```python
from build123d import *

# Parameters (mm, degrees)
F1_DEPTH = 609.6
F2_R     = 12.7
F3_DEPTH = 406.401
F4_T     = -2.54
F5_R     = 12.7
F5_R_2   = 3.302
F6_DEPTH = 25.4


with BuildPart() as f1:
    # F0 (on Top) → F1 (new body)
    with BuildSketch(Plane.XY):
        with BuildLine():
            Line((203.2, -101.6), (203.2, 114.3))
            Line((203.2, 114.3), (-203.2, 114.3))
            Line((-203.2, 114.3), (-203.2, -101.6))
            ThreePointArc((-203.2, -101.6), (-194.2197438789, -105.3197438789), (-190.5, -114.3))
            Line((-190.5, -114.3), (190.5, -114.3))
            ThreePointArc((190.5, -114.3), (194.2197438789, -105.3197438789), (203.2, -101.6))
        make_face()
    extrude(amount=F1_DEPTH)

    # F2 (on face) → F3 (cut, through all)
    with BuildSketch(Plane.YZ.offset(203.2)):
        with Locations((-114.2978898402, 609.8315029268)):
            Circle(F2_R)
        with Locations((-114.3, 0)):
            Circle(F2_R)
    extrude(amount=-F3_DEPTH, mode=Mode.SUBTRACT)

    # F4
    f4_openings = [f1.faces().sort_by_distance(p)[0] for p in [
        (0, -114.3, 304.915752),
    ]]
    offset(amount=F4_T, openings=f4_openings)

    # F5 (on face) → F6 (cut)
    with BuildSketch(Plane.XY.offset(609.6)):
        with Locations((127, 25.4)):
            Circle(F5_R)
        with Locations((101.6, 25.4)):
            Circle(F5_R_2)
    extrude(amount=-F6_DEPTH, mode=Mode.SUBTRACT)


solid = f1.part
```
CAD build for the part. Positions are in the model's coordinates, mm. A direction names the side the tool comes from. Coordinates: 2 decimals unless noted, no trailing zeros. Loops run counter-clockwise (first coordinate to the right, second up) from the corner with the lowest first, then second, coordinate; pieces in that order, holes last. Notation, with made-up numbers: (49.25, -4) - (54.25, -4) arc R28 ccw to (54.25, 23) - close; hole circle Ø5 at (33.25, 79.5). An arc over 180 degrees is marked (long way). Return JSON: item names as keys, results as strings.
1. Probe L1, parallel to X at y = 25, z = 608; L2, parallel to Z at x = 180, y = -8; L3, parallel to X at y = 25, z = 607. List the from-to ranges inside material, lowest first. Write a range as from..to.
Result:
{"L1": "x = -203.2..98.32, 104.88..114.31, 139.69..203.2", "L2": "z = 0..2.54, 607.06..609.6", "L3": "x = -203.2..-200.66, 200.66..203.2"}
2. Mould opens along Z. For faces 4 (the cylindrical face through (2.81, -104.67, 598.02)), 5 (the flat face through (203.2, 5, 301)), 6 (the cylindrical face through (2.84, -105.5, 600.67)), 7 (the cylindrical face through (2.84, -105.22, 8.88)) say: released by +Z, released by -Z, zero draft, split by the parting line, or undercut.
Result:
{"face 4": "undercut", "face 5": "zero draft", "face 6": "released by +Z", "face 7": "released by -Z"}
3. Drop a flat-ended pin along its axis: pin 1 (3 mm diameter, centred on x = -145.5, z = 372.5, fed in from -Y). Give the stop position or say it passes through.
Result:
{"pin 1": "stops at y = 111.76"}
4. Band-saw the part on C-C (z = 295.5). Give the cut face in (x, y).
Result:
{"outline": "(-203.2, -101.6) arc R12.7 cw to (-190.5, -114.3) - (-187.96, -114.3) arc R15.24 ccw to (-200.66, -99.27) - (-200.66, 111.76) - (200.66, 111.76) - (200.66, -99.27) arc R15.24 ccw to (187.96, -114.3) - (190.5, -114.3) arc R12.7 cw to (203.2, -101.6) - (203.2, 114.3) - (-203.2, 114.3) - close"}
5. Band-saw the part on D-D (x = -96.5). Give the cut face in (y, z), and give its area (3 significant figures).
Result:
{"outline": "(-114.3, 12.7) arc R12.7 cw to (-101.6, 0) - (114.3, 0) - (114.3, 609.6) - (-101.6, 609.6) arc R12.7 cw to (-114.3, 597.13) - (-114.3, 594.59) arc R15.24 ccw to (-99.31, 607.06) - (111.76, 607.06) - (111.76, 2.54) - (-99.27, 2.54) arc R15.24 ccw to (-114.3, 15.24) - close", "area": "2,730 mm2"}
6. 3-axis set-ups, long thin cutter, end or side, ignore diameter. For faces 1 (the cylindrical face through (-191.7, -104.3, 300.6)), 2 (the flat face through (-203.2, 8, 301)), 3 (the cylindrical face through (133.827, 36.109, 608.348)): which of +Z, -Z, +X, -X, +Y, -Y reach the whole face in a straight line?
Result:
{"face 1": "none", "face 2": "+Z, -Z, -X, +Y, -Y", "face 3": "+Z"}
7. Band-saw the part on B-B (x = 127). Give the cut face in (y, z), and give its area (3 significant figures).
Result:
{"outline": "(-114.3, 12.7) arc R12.7 cw to (-101.6, 0) - (114.3, 0) - (114.3, 609.6) - (38.1, 609.6) - (38.1, 607.06) - (111.76, 607.06) - (111.76, 2.54) - (-99.27, 2.54) arc R15.24 ccw to (-114.3, 15.24) - close; (-114.3, 594.59) arc R15.24 ccw to (-99.31, 607.06) - (12.7, 607.06) - (12.7, 609.6) - (-101.6, 609.6) arc R12.7 cw to (-114.3, 597.13) - close", "area": "2,670 mm2"}
8. Band-saw the part on A-A (y = -11.5). Give the cut face in (x, z), and give its area (3 significant figures).
Result:
{"outline": "(-203.2, 0) - (203.2, 0) - (203.2, 609.6) - (-203.2, 609.6) - close; hole (-200.66, 2.54) - (200.66, 2.54) - (200.66, 607.06) - (-200.66, 607.06) - close", "area": "5,140 mm2"}
